```python
from build123d import *

# Parameters (mm, degrees)
SKETCH1_R           = 9.5
BOSS_EXTRUDE1_DEPTH = 10
BOSS_EXTRUDE4_START = -9.75
BOSS_EXTRUDE4_DEPTH = 9.75
BOSS_EXTRUDE5_DEPTH = 9.75
SKETCH19_R          = 2.675
CUT_EXTRUDE1_DEPTH  = 54.237071403
CUT_EXTRUDE2_DEPTH  = 1
SKETCH21_R          = 9.541498329
BOSS_EXTRUDE6_DEPTH = 8
SKETCH22_W          = 10.184582577
SKETCH22_H          = 8
CUT_EXTRUDE3_DEPTH  = 1
SKETCH24_R          = 2.6
BOSS_EXTRUDE8_DEPTH = 1
SKETCH25_R          = 2.6
BOSS_EXTRUDE9_DEPTH = 5
SKETCH26_R          = 4.5
CUT_EXTRUDE4_DEPTH  = 5
CUT_EXTRUDE5_DEPTH  = 5
FILLET1_R           = 3
FILLET2_R           = 10


with BuildPart() as part:
    # Sketch1 → Boss-Extrude1 (new body)
    with BuildSketch(Plane.XY):
        with BuildLine():
            Line((-23.433441641, -14.957015859), (-23.433441641, -24.707015859))
            Line((-23.433441641, -24.707015859), (14.870192677, -24.707015859))
            ThreePointArc((14.870192677, -24.707015859), (18.975681404, -23.376668609), (21.520677092, -19.891290805))
            Line((21.520677092, -19.891290805), (25.525569024, -7.69755511))
            ThreePointArc((25.525569024, -7.69755511), (26.630542081, -2.207015859), (25.525569024, 3.283523393))
            Line((25.525569024, 3.283523393), (21.520677092, 15.477259087))
            ThreePointArc((21.520677092, 15.477259087), (18.975681404, 18.962636892), (14.870192677, 20.292984141))
            Line((14.870192677, 20.292984141), (-23.433441641, 20.292984141))
            Line((-23.433441641, 20.292984141), (-23.433441641, 10.542984141))
            Line((-23.433441641, 10.542984141), (-3.433441641, 10.542984141))
            Line((-3.433441641, 10.542984141), (-3.433441641, 1.794523598))
            Line((-3.433441641, 1.794523598), (-1.933441641, 1.794523598))
            Line((-1.933441641, 1.794523598), (-1.933441641, -6.205476402))
            Line((-1.933441641, -6.205476402), (-3.433441641, -6.205476402))
            Line((-3.433441641, -6.205476402), (-3.433441641, -14.957015859))
            Line((-3.433441641, -14.957015859), (-23.433441641, -14.957015859))
        make_face()
        with Locations((12.436989349, -2.207015859)):
            Circle(SKETCH1_R, mode=Mode.SUBTRACT)
        Polygon((10.026551975, -12.925000001), (14.847426723, -12.925000001), (17.257864097, -17.100000001), (14.847426723, -21.275000001), (10.026551975, -21.275000001), (7.616114601, -17.100000001), align=None, mode=Mode.SUBTRACT)
        Polygon((14.847426723, 8.724999999), (17.257864097, 12.899999999), (14.847426723, 17.074999999), (10.026551975, 17.074999999), (7.616114601, 12.899999999), (10.026551975, 8.724999999), align=None, mode=Mode.SUBTRACT)
    extrude(amount=BOSS_EXTRUDE1_DEPTH)

    # Sketch2 → Boss-Extrude4 (add)
    with BuildSketch(Plane(origin=(0, 20.292984141, 0), x_dir=(1, 0, 0), z_dir=(0, 1, 0)).offset(BOSS_EXTRUDE4_START)):
        with BuildLine():
            Line((-23.433441641, 0), (-3.433441641, 0))
            ThreePointArc((-3.433441641, 0), (-6.362373829, 7.071067812), (-13.433441641, 10))
            Line((-13.433441641, 10), (-23.433441641, 10))
            Line((-23.433441641, 10), (-23.433441641, 0))
        make_face()
    extrude(amount=BOSS_EXTRUDE4_DEPTH)

    # Sketch18 → Boss-Extrude5 (add)
    with BuildSketch(Plane.XZ.offset(24.707015859)):
        with BuildLine():
            Line((-23.433441641, 0), (-3.433441641, 0))
            ThreePointArc((-3.433441641, 0), (-6.362373829, -7.071067812), (-13.433441641, -10))
            Line((-13.433441641, -10), (-23.433441641, -10))
            Line((-23.433441641, -10), (-23.433441641, 0))
        make_face()
    extrude(amount=-BOSS_EXTRUDE5_DEPTH)

    # Sketch19 → Cut-Extrude1 (cut, through all)
    with BuildSketch(Plane.XZ.offset(24.707015859)):
        with Locations(Location((-13.433441641, 0, 0), (0, 0, 270))):
            Circle(SKETCH19_R)
    extrude(amount=-CUT_EXTRUDE1_DEPTH, mode=Mode.SUBTRACT)

    # Sketch20 → Cut-Extrude2 (cut)
    with BuildSketch(Plane(origin=(0, 0, 0), x_dir=(-1, 0, 0), z_dir=(0, 0, -1))):
        Polygon((3.433441641, -24.707015859), (3.433441641, 20.292984141), (-35.58098809, 20.292984141), (-33.558086905, -24.707015859), align=None)
    extrude(amount=-CUT_EXTRUDE2_DEPTH, mode=Mode.SUBTRACT)

    # Sketch21 → Boss-Extrude6 (add)
    with BuildSketch(Plane.XY.offset(10)):
        with Locations((12.436989349, -2.207015859)):
            Circle(SKETCH21_R)
    extrude(amount=-BOSS_EXTRUDE6_DEPTH)

    # Sketch22 → Cut-Extrude3 (cut)
    with BuildSketch(Plane(origin=(0, 0, 1), x_dir=(-1, 0, 0), z_dir=(0, 0, -1))):
        with Locations((-3.158849648, -2.205476402)):
            Rectangle(SKETCH22_W, SKETCH22_H)
    extrude(amount=-CUT_EXTRUDE3_DEPTH, mode=Mode.SUBTRACT)

    # Sketch24 → Boss-Extrude8 (add)
    # profile 1 of 3: a face of its own
    with BuildSketch(Plane.XY.offset(10)):
        with BuildLine():
            Line((14.870192677, -24.707015859), (-23.433441641, -24.707015859))
            Line((-23.433441641, -24.707015859), (-23.433441641, -14.957015859))
            Line((-23.433441641, -14.957015859), (-3.433441641, -14.957015859))
            Line((-3.433441641, -14.957015859), (-3.433441641, -6.205476402))
            Line((-3.433441641, -6.205476402), (-1.933441641, -6.205476402))
            Line((-1.933441641, -6.205476402), (-1.933441641, 1.794523598))
            Line((-1.933441641, 1.794523598), (-3.433441641, 1.794523598))
            Line((-3.433441641, 1.794523598), (-3.433441641, 10.542984141))
            Line((-3.433441641, 10.542984141), (-23.433441641, 10.542984141))
            Line((-23.433441641, 10.542984141), (-23.433441641, 20.292984141))
            Line((-23.433441641, 20.292984141), (14.870192677, 20.292984141))
            ThreePointArc((14.870192677, 20.292984141), (18.975681404, 18.962636892), (21.520677092, 15.477259087))
            Line((21.520677092, 15.477259087), (25.525569024, 3.283523393))
            ThreePointArc((25.525569024, 3.283523393), (26.630542081, -2.207015859), (25.525569024, -7.69755511))
            Line((25.525569024, -7.69755511), (21.520677092, -19.891290805))
            ThreePointArc((21.520677092, -19.891290805), (18.975681404, -23.376668609), (14.870192677, -24.707015859))
        make_face()
        Polygon((14.847426723, 8.724999999), (17.257864097, 12.899999999), (14.847426723, 17.074999999), (10.026551975, 17.074999999), (7.616114601, 12.899999999), (10.026551975, 8.724999999), align=None, mode=Mode.SUBTRACT)
        Polygon((10.026551975, -12.925000001), (14.847426723, -12.925000001), (17.257864097, -17.100000001), (14.847426723, -21.275000001), (10.026551975, -21.275000001), (7.616114601, -17.100000001), align=None, mode=Mode.SUBTRACT)
    # profile 2 of 3: a face of its own
    with BuildSketch(Plane.XY.offset(10)):
        with Locations((12.436989349, 12.899999999)):
            Circle(SKETCH24_R)
    # profile 3 of 3: a face of its own
    with BuildSketch(Plane.XY.offset(10)):
        with Locations((12.436989349, -17.100000001)):
            Circle(SKETCH24_R)
    extrude(amount=BOSS_EXTRUDE8_DEPTH)


with BuildPart() as boss_extrude8_kept_piece:
    # of the separate pieces the step leaves, the one the design keeps (boss_extrude8_pieces_kept)
    add(part.part.solids().sort_by_distance((-3.433441641, -14.957015859, 0))[0])

    # Sketch25 → Boss-Extrude9 (add)
    # profile 1 of 2: a face of its own
    with BuildSketch(Plane.XY.offset(11)):
        Polygon((10.026551975, 8.724999999), (14.847426723, 8.724999999), (17.257864097, 12.899999999), (14.847426723, 17.074999999), (10.026551975, 17.074999999), (7.616114601, 12.899999999), align=None)
        with Locations((12.436989349, 12.899999999)):
            Circle(SKETCH25_R, mode=Mode.SUBTRACT)
    # profile 2 of 2: a face of its own
    with BuildSketch(Plane.XY.offset(11)):
        Polygon((14.847426723, -12.925000001), (10.026551975, -12.925000001), (7.616114601, -17.100000001), (10.026551975, -21.275000001), (14.847426723, -21.275000001), (17.257864097, -17.100000001), align=None)
        with Locations((12.436989349, -17.100000001)):
            Circle(SKETCH25_R, mode=Mode.SUBTRACT)
    extrude(amount=-BOSS_EXTRUDE9_DEPTH)

    # Sketch26 → Cut-Extrude4 (cut)
    with BuildSketch(Plane.XZ.offset(24.707015859)):
        with Locations((-13.433441641, 0)):
            Circle(SKETCH26_R)
    extrude(amount=-CUT_EXTRUDE4_DEPTH, mode=Mode.SUBTRACT)

    # Sketch27 → Cut-Extrude5 (cut)
    with BuildSketch(Plane(origin=(0, 20.292984141, 0), x_dir=(1, 0, 0), z_dir=(0, 1, 0))):
        Polygon((-8.612566893, 0), (-11.023004267, 4.175), (-15.843879015, 4.175), (-18.254316389, 0), (-15.843879015, -4.175), (-11.023004267, -4.175), align=None)
    extrude(amount=-CUT_EXTRUDE5_DEPTH, mode=Mode.SUBTRACT)

    # Fillet1
    fillet1_edges = [boss_extrude8_kept_piece.edges().sort_by_distance(p)[0] for p in [
        (-1.933441641, -2.205476402, 2),
    ]]
    fillet(fillet1_edges, radius=FILLET1_R)

    # Fillet2
    fillet2_edges = [boss_extrude8_kept_piece.edges().sort_by_distance(p)[0] for p in [
        (-23.433441641, -19.832015859, -10),
        (-23.433441641, 15.417984141, -10),
    ]]
    fillet(fillet2_edges, radius=FILLET2_R - 0.0001)  # a hair under: the kernel refuses the full size


solid = boss_extrude8_kept_piece.part
```
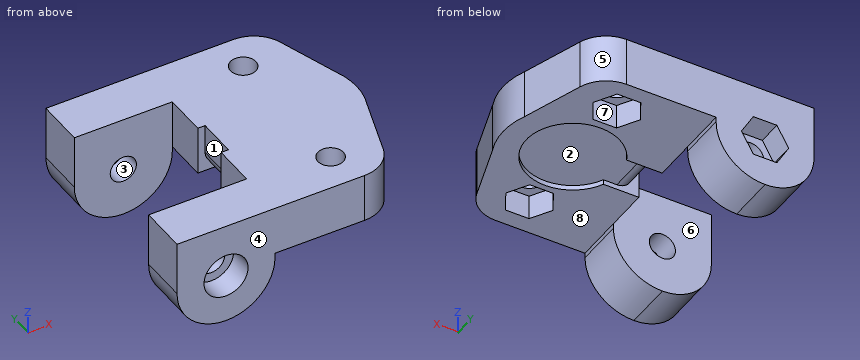
Could you check a few things on this model? Use its own coordinates, in mm. Face numbers are marked on the shaded views. A direction names the side the tool comes from. Give positions to 0.01 mm unless a question says otherwise; leave off trailing zeros. Loops run counter-clockwise (first coordinate to the right, second up) from the corner with the lowest first, then second, coordinate; pieces in that order, holes last. Notation, with made-up numbers: (-19, -6) -> (20, -6) arc R32 cw to (20, 28) -> close; hole circle Ø8 at (60.25, 30.5). An arc over 180 degrees is marked (long way). Put each result on its own line as item: value.
(1) Thinking about a two-plate mould opening in X: for the marked faces 1, 2, 3 and 4, which applies, pulls with the +X half, pulls with the -X half, needs draft (parallel to the pull), parting line crosses it, or undercut?
Computed:
face 1: pulls with the -X half
face 2: undercut
face 3: undercut
face 4: needs draft
(2) Imagine slicing it at D-D on x = -20. Write out the boundary of the cut face in (y, z), plus the area to 3 significant figures.
Computed:
outline: (-24.71, -7.54) -> (-14.96, -7.54) -> (-14.96, 11) -> (-24.71, 11) -> close; (10.54, -7.54) -> (20.29, -7.54) -> (20.29, 11) -> (10.54, 11) -> close
area: 362 mm^2
(3) Imagine slicing it at C-C on y = -3. Write out the boundary of the cut face in (x, z), plus the area to 3 significant figures.
Computed:
outline: (-1.93, 5) arc R3 ccw to (1.07, 2) -> (21.9, 2) -> (21.9, 1) -> (26.61, 1) -> (26.61, 11) -> (-1.93, 11) -> close
area: 260 mm^2
(4) Imagine slicing it at A-A on x = 14. Write out the boundary of the cut face in (y, z) (3 decimals).
Computed:
outline: (-24.707, 1) -> (-21.275, 1) -> (-21.275, 6) -> (-19.178, 6) -> (-19.178, 11) -> (-24.707, 11) -> close; (-15.022, 6) -> (-12.925, 6) -> (-12.925, 1) -> (-11.578, 1) -> (-11.578, 2) -> (7.164, 2) -> (7.164, 1) -> (8.725, 1) -> (8.725, 6) -> (10.822, 6) -> (10.822, 11) -> (-15.022, 11) -> close; (14.978, 6) -> (17.075, 6) -> (17.075, 1) -> (20.293, 1) -> (20.293, 11) -> (14.978, 11) -> close
(5) For the marked faces 5, 6, 7 and 8, which set-ups out of +Z, -Z, +X, -X, +Y, -Y let a thin tool reach every point of the face, with its end or its side?
Computed:
face 5: +Z, -Z, +X, +Y
face 6: +Z, -Z, -X
face 7: -Z
face 8: -Z, +X, +Y, -Y
(6) Imagine slicing it at B-B on z = -7.25. Write out the boundary of the cut face in (x, y).
Computed:
outline: (-20.32, -24.71) -> (-6.55, -24.71) -> (-6.55, -14.96) -> (-20.32, -14.96) -> close; (-20.32, 10.54) -> (-6.55, 10.54) -> (-6.55, 20.29) -> (-20.32, 20.29) -> close
(7) I'm going to push flat-ended pins straight in: pin 1 Ø9 at (x, y) = (10.5, 14.5) entering from -Z; pin 2 Ø7 at (x, y) = (12.44, 12.9) entering from -Z; pin 3 Ø10 at (x, y) = (-8, -11) entering from -Z; pin 4 Ø7 at (x, z) = (-14.5, -1) entering from -Y. Where does each tip first touch, or does it pass through?
Computed:
pin 1: z = 1
pin 2: z = 6
pin 3: z = -9.71
pin 4: y = -24.71
(8) Please list where these lines run through material, in increasing order: probe 1 along Y at (x, z) = (-7, 0.75); probe 2 along Y at (x, z) = (-10, -2); probe 3 along Y at (x, z) = (12, 1.5) (3 decimals). Write a range as [from, to].
Computed:
probe 1: [-24.71, -14.96], [10.54, 20.29]
probe 2: [-19.71, -14.96], [10.54, 15.29]
probe 3: [-24.707, -21.275], [-12.925, -11.697], [7.283, 8.725], [17.075, 20.293]
